Geometry: see drawing. Coordinates: mm, zero at the bounding-box minimum. A direction names the side the tool comes from. Coordinates: 2 decimals unless noted, no trailing zeros. Order: outer loops, then holes, each group sorted by start corner. A loop starts at its lowest first (then second) coordinate and runs counter-clockwise, first axis right, second up. Notation, with made-up numbers: M 60.5,73 L 80.5,73 A7 ccw 80.5,83 Z; hole C 59.5,85 d9. An arc over 180 degrees is marked long. Answer in a Markdown table with one row per item.
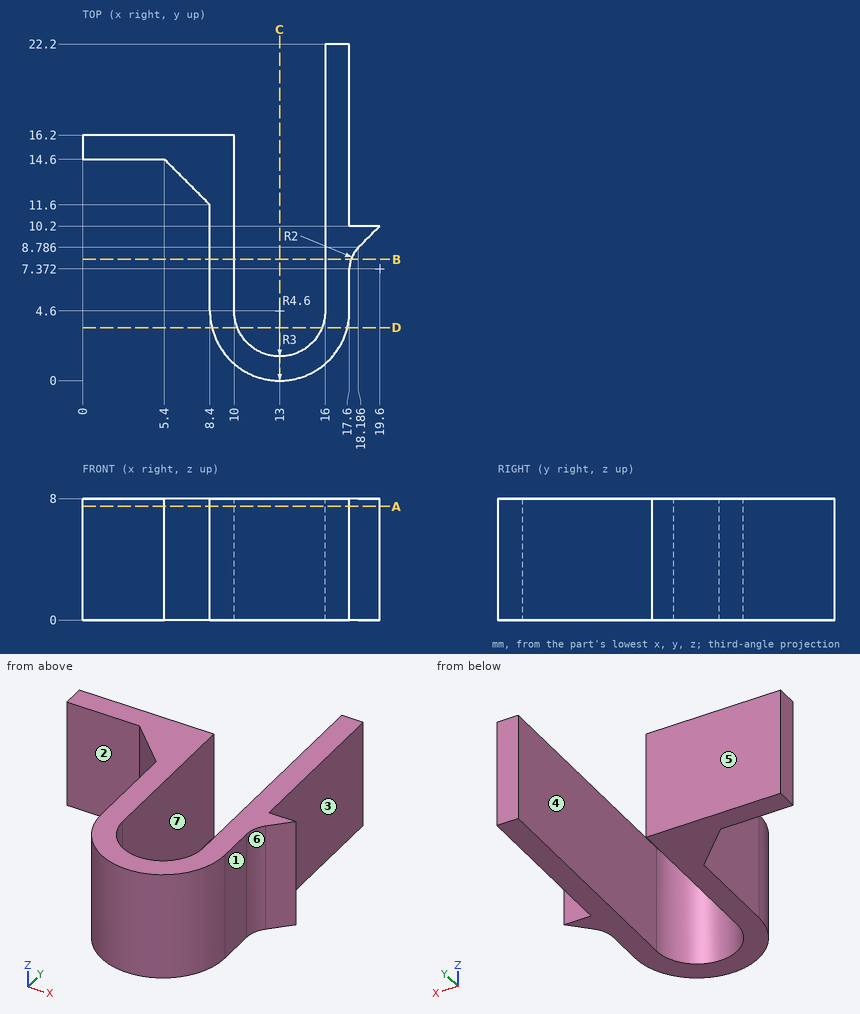
1) Cut plane B-B, the plane y = 8. Output: boundary loops of the cut face in (x, z), and give its area (3 significant figures).
Resolved:
| item | result |
|---|---|
| outline | M 8.4,0 L 10,0 L 10,8 L 8.4,8 Z; M 16,0 L 17.7,0 L 17.7,8 L 16,8 Z |
| area | 26.4 mm2 |
2) Mould query, pull axis X, two halves, no side actions, for the marked faces 5, 6 and 7. Classes: +X half, -X half, draft (parallel to the pull), parting line (faces both ways), or undercut.
Resolved:
| item | result |
|---|---|
| face 5 | draft |
| face 6 | +X half |
| face 7 | undercut |
3) Reachability of the marked faces 1, 2, 3 and 4 from +Z, -Z, +X, -X, +Y, -Y: full face, straight path, thin tool, end or side. Return the list, or none.
Resolved:
| item | result |
|---|---|
| face 1 | +Z, -Z, +X, -Y |
| face 2 | +Z, -Z, -X, -Y |
| face 3 | +Z, -Z, +X, +Y |
| face 4 | +Z, -Z, +Y |
4) Cut plane C-C, the plane x = 13. Output: boundary loops of the cut face in (y, z).
Resolved:
| item | result |
|---|---|
| outline | M 0,0 L 1.6,0 L 1.6,8 L 0,8 Z |
5) Material intervals for probe 1 along X at (y, z) = (15, 4.5); probe 2 along X at (y, z) = (11.5, 6.25); probe 3 along X at (y, z) = (16.5, 6.5), sorted ascending.
Resolved:
| item | result |
|---|---|
| probe 1 | x = 0 to 10, 16 to 17.6 |
| probe 2 | x = 8.4 to 10, 16 to 17.6 |
| probe 3 | x = 16 to 17.6 |
6) Cut plane A-A, the plane z = 7.5. Output: boundary loops of the cut face in (x, y) (1 decimal).
Resolved:
| item | result |
|---|---|
| outline | M 0,14.6 L 5.4,14.6 L 8.4,11.6 L 8.4,4.6 A4.6 ccw 17.6,4.6 L 17.6,7.4 A2 cw 18.2,8.8 L 19.6,10.2 L 17.6,10.2 L 17.6,22.2 L 16,22.2 L 16,4.6 A3 cw 10,4.6 L 10,16.2 L 0,16.2 Z |
7) Contact query for flat-ended pins moving along their axis: pin 1 (4.5 mm diameter, centred on x = 3, z = 6, fed in from -Y); pin 2 (3 mm diameter, centred on y = 12.5, z = 5, fed in from +X); pin 3 (3 mm diameter, centred on y = 6.5, z = 5.5, fed in from +X). Output: stop coordinate, or through.
Resolved:
| item | result |
|---|---|
| pin 1 | stops at y = 14.6 |
| pin 2 | stops at x = 17.6 |
| pin 3 | stops at x = 17.7 |
8) Cut plane D-D, the plane y = 3.5. Output: boundary loops of the cut face in (x, z).
Resolved:
| item | result |
|---|---|
| outline | M 8.53,0 L 10.21,0 L 10.21,8 L 8.53,8 Z; M 15.79,0 L 17.47,0 L 17.47,8 L 15.79,8 Z |
